Autodesk Inventor part; units mm, degrees
ref_plane "YZ Plane" through (0, 0, 0) normal (1, 0, 0) x (0, 1, 0)
ref_plane "XZ Plane" through (0, 0, 0) normal (0, 1, 0) x (-1, 0, 0)
ref_plane "XY Plane" through (0, 0, 0) normal (0, 0, 1) x (1, 0, 0)
sketch "Sketch1" plane through (0, 0, 0) normal (0, 0, 1) x (1, 0, 0)
  circle A0 centre (0, 0) radius 5.75
  dimension "d0" = 11.5
extrude "Extrusion1" add sketch "Sketch1" along normal blind 1.5
fillet "Fillet1" radius 1.5 1 edges at (-5.75, 0, 1.5)
sketch "Sketch2" plane through (0, 0, 1.5) normal (0, 0, 1) x (1, 0, 0)
  circle A0 centre (0, 0) radius 1.65
  dimension "d4" = 3.3
extrude "Extrusion2" cut sketch "Sketch2" against normal blind 1.5
sketch "Sketch3" plane through (0, 0, 0) normal (0, 0, -1) x (-1, 0, 0)
  circle A0 centre (0, 0) radius 1.65
  circle A1 centre (0, 0) radius 5.75
  circle A2 centre (0, 0) radius 3.25
  dimension "d7" = 6.5
extrude "Extrusion3" cut sketch "Sketch3" against normal blind 1 contours A2
properties part number "Spacer_Top_Plate_Bearing"
Design review of the part built by this model. Coordinates are the model's own, in mm. A direction names the side the tool comes from. Coordinates: 2 decimals unless noted, no trailing zeros. Order: outer loops, then holes, each group sorted by start corner. A loop starts at its lowest first (then second) coordinate and runs counter-clockwise, first axis right, second up.
Item 1: Take a section at C-C, the plane z = 0.45. Write out the cut boundary in (x, y), then the cut area to 3 significant figures.
Item 2: For pin 1 Ø2 at (x, y) = (1, 1) entering from -Z, flat-tipped, find the tip position at first contact; note if it passes through.
Item 3: The part is to be moulded in two halves that separate along X. For faces 3 (the cylindrical face through (2.579, -1.978, 0.493)), 4 (the flat face through (0, -2, 1.5)), 5 (the cylindrical face through (-1.216, 1.115, 1.254)), say which applies: pulls with the +X half, pulls with the -X half, needs draft (parallel to the pull), parting line crosses it, or undercut.
Item 4: For line 1 (Y direction, x = 0.25, z = 0.95); line 2 (Y direction, x = 0.75, z = 0.45); line 3 (X direction, y = 2.5, z = 0.1), list the stretches that pass through material, from the lowest coordinate up.
Item 5: For faces 1 (the flat face through (2.5, -2.5, 0)), 2 (the flat face through (-1.4, -1.4, 1)), list the 3-axis set-ups (+Z, -Z, +X, -X, +Y, -Y) from which the entire face can be reached by the end or side of a thin tool; tool diameter is ignored.
Item 6: Take a section at D-D, the plane z = 1.35. Write out the cut boundary in (x, y).
The answers:
1. outline: circle Ø11.36 at (0, 0); hole circle Ø6.5 at (0, 0)
1. area: 68.2 mm2
2. pin 1: stops at z = 1
3. face 3: undercut
3. face 4: needs draft
3. face 5: undercut
4. line 1: y = -5.41 to -3.24, 3.24 to 5.41
4. line 2: y = -5.63 to -3.16, 3.16 to 5.63
4. line 3: x = -5.17 to -2.08, 2.08 to 5.17
5. face 1: -Z, +X, -X, +Y, -Y
5. face 2: -Z
6. outline: circle Ø9.81 at (0, 0); hole circle Ø3.3 at (0, 0)
